Source: three-view drawing plus pictorial views. Frame: mm from the lowest corner of the part. A direction names the side the tool comes from. Round coordinates to 2 decimals unless told otherwise and drop trailing zeros. Loops run counter-clockwise (first coordinate to the right, second up) from the corner with the lowest first, then second, coordinate; pieces in that order, holes last. Notation, with made-up numbers: (-37.75, 5) -> (19.25, 5) arc R30 ccw to (19.25, 40) -> close; hole circle Ø2 at (12.5, 57). An arc over 180 degrees is marked (long way). Answer in a Markdown table with one row per item.
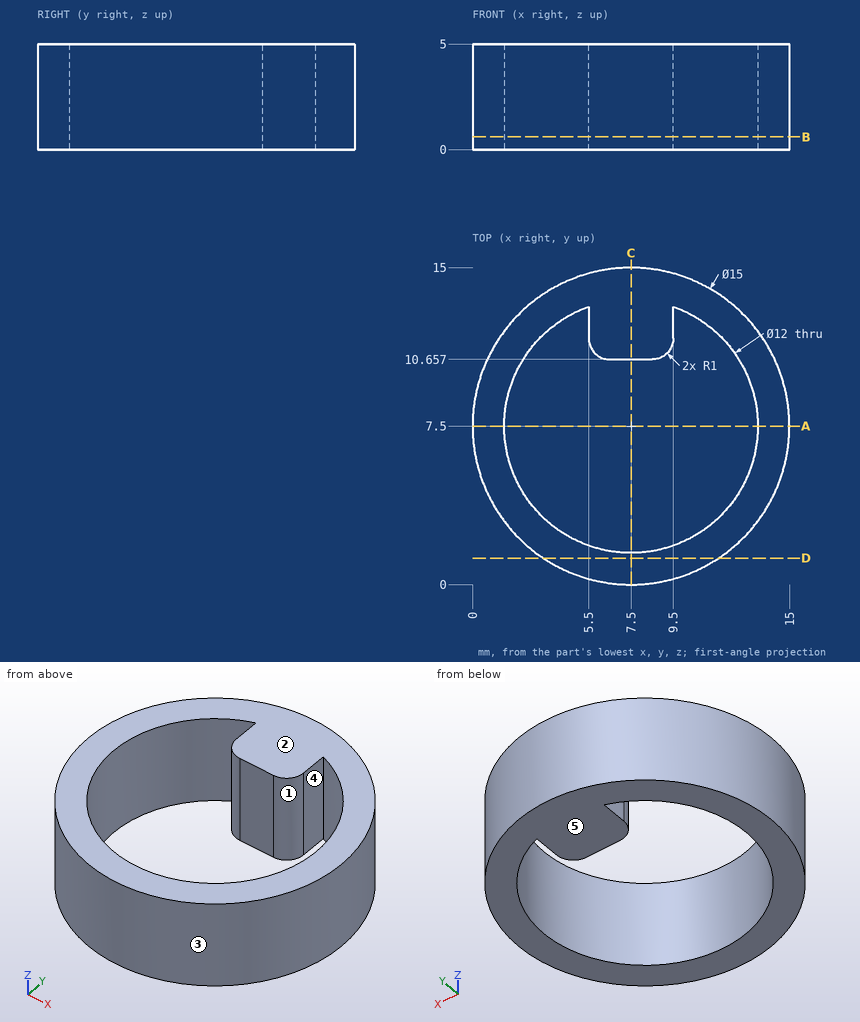
Item 1: Cut plane D-D (y = 1.25). Output: boundary loops of the cut face in (x, z).
Answer:
| item | result |
|---|---|
| outline | (3.35, 0) -> (11.65, 0) -> (11.65, 5) -> (3.35, 5) -> close |
Item 2: Pin query (flat end, axial travel): pin 1 Ø1.5 at (y, z) = (4.5, 1.5) entering from +X; pin 2 Ø1.5 at (x, y) = (3, 4) entering from +Z; pin 3 Ø3 at (x, z) = (10, 1) entering from -Y; pin 4 Ø1.7 at (y, z) = (12.5, 3.5) entering from -X. Return the tip coordinate at first contact, or that it passes through.
Answer:
| item | result |
|---|---|
| pin 1 | stops at x = 14.65 |
| pin 2 | stops at z = 5 |
| pin 3 | stops at y = 0.07 |
| pin 4 | stops at x = 1.25 |
Item 3: Reachability of the marked faces 1 and 2 from +Z, -Z, +X, -X, +Y, -Y: full face, straight path, thin tool, end or side. Return the list, or none.
Answer:
| item | result |
|---|---|
| face 1 | +Z, -Z |
| face 2 | +Z, +X, -X, +Y, -Y |
Item 4: Cut plane C-C (x = 7.5). Output: boundary loops of the cut face in (y, z).
Answer:
| item | result |
|---|---|
| outline | (0, 0) -> (1.5, 0) -> (1.5, 5) -> (0, 5) -> close; (10.66, 0) -> (15, 0) -> (15, 5) -> (10.66, 5) -> close |
Item 5: Cut plane B-B (z = 0.6). Output: boundary loops of the cut face in (x, y), then the cut area to 3 significant figures.
Answer:
| item | result |
|---|---|
| outline | circle Ø15 at (7.5, 7.5); hole (5.5, 11.66) -> (5.5, 13.16) arc R6 ccw (long way) to (9.5, 13.16) -> (9.5, 11.66) arc R1 cw to (8.5, 10.66) -> (6.5, 10.66) arc R1 cw to start |
| area | 74.1 mm² |
Item 6: Draft query along X for the marked faces 3, 4 and 5. Return one class per face: pulls with the +X half, pulls with the -X half, needs draft (parallel to the pull), parting line crosses it, or undercut.
Answer:
| item | result |
|---|---|
| face 3 | parting line crosses it |
| face 4 | undercut |
| face 5 | needs draft |
Item 7: Line query: probe 1 along Y at (x, z) = (7.5, 2.6); probe 2 along X at (y, z) = (12.5, 4.15); probe 3 along Y at (x, z) = (4.75, 1.3). Output: solid intervals per line, ascending. Write a range as [from, to].
Answer:
| item | result |
|---|---|
| probe 1 | y = [0, 1.5], [10.66, 15] |
| probe 2 | x = [1.91, 4.18], [5.5, 9.5], [10.82, 13.09] |
| probe 3 | y = [0.52, 2.17], [12.83, 14.48] |
Item 8: Cut plane A-A (y = 7.5). Output: boundary loops of the cut face in (x, z).
Answer:
| item | result |
|---|---|
| outline | (0, 0) -> (1.5, 0) -> (1.5, 5) -> (0, 5) -> close; (13.5, 0) -> (15, 0) -> (15, 5) -> (13.5, 5) -> close |
